```python
from build123d import *

# Parameters (mm, degrees)
SWEEP3_PROFILE_R    = 3.1
SKETCH17_R          = 4.95
BOSS_EXTRUDE1_DEPTH = 15
SKETCH18_R          = 3.85
BOSS_EXTRUDE2_DEPTH = 5
SKETCH19_R          = 4.95
BOSS_EXTRUDE3_DEPTH = 15
SKETCH20_R          = 3.85
BOSS_EXTRUDE4_DEPTH = 5


with BuildPart() as part:
    # Sweep3: sweep along a path in Sketch9
    with BuildLine(Plane.XY) as sweep3_path:
        Line((-183.399133976, 40), (-183.399133976, 180))
        ThreePointArc((-183.399133976, 180), (-130.108654619, 241.593132461), (-61.492979679, 197.712860026))
    # Sweep3 profile (on start of the path) → Sweep3 (sweep)
    with BuildSketch(Plane(origin=(-183.399133976, 40, 0), x_dir=(0, 0, 1), z_dir=(0, 1, 0))):
        Circle(SWEEP3_PROFILE_R)
    sweep(path=sweep3_path.line)

    # Sketch17 → Boss-Extrude1 (add)
    with BuildSketch(Plane.XZ.offset(-40)):
        with Locations((-183.399133976, 0)):
            Circle(SKETCH17_R)
    extrude(amount=BOSS_EXTRUDE1_DEPTH)

    # Sketch18 → Boss-Extrude2 (add)
    with BuildSketch(Plane.XZ.offset(-25)):
        with Locations((-183.399133976, 0)):
            Circle(SKETCH18_R)
    extrude(amount=BOSS_EXTRUDE2_DEPTH)

    # Sketch19 → Boss-Extrude3 (add)
    with BuildSketch(Plane(origin=(-58.920841531, 198.476439545, 0), x_dir=(0.9586493060523679, 0.28459007011017384, 0), z_dir=(0.2845900701101738, -0.9586493060523678, 0))):
        with Locations(Location((-2.6830856, 0, 0), (0, 0, 180))):
            Circle(SKETCH19_R)
    extrude(amount=BOSS_EXTRUDE3_DEPTH)

    # Sketch20 → Boss-Extrude4 (add)
    with BuildSketch(Plane(origin=(-54.651990479, 184.096699954, 0), x_dir=(0.9586493060523679, 0.2845900701101739, 0), z_dir=(0.28459007011017384, -0.9586493060523678, 0))):
        with Locations(Location((-2.6830856, 0, 0), (0, 0, 180))):
            Circle(SKETCH20_R)
    extrude(amount=BOSS_EXTRUDE4_DEPTH)


solid = part.part
```
Here's how the part is built. I have some questions about the finished solid (model axes, mm). A direction names the side the tool comes from. Coordinates: 2 decimals unless noted, no trailing zeros. Order: outer loops, then holes, each group sorted by start corner. A loop starts at its lowest first (then second) coordinate and runs counter-clockwise, first axis right, second up. Notation, with made-up numbers: M -13.75,46.25 L 5.25,46.25 A21 cw 5.25,77.25 Z; hole C -3,-17.5 d3. An arc over 180 degrees is marked long. Answer as a JSON object with one key per item and string values. Group by question number.
(1) If we mould it in two halves opening along X, with no side actions, what happens to faces 1 (the face through (-52.835, 182.065, -0.169)), 2 (the face through (-183, 20, 0)), 3 (the face through (-187.245, 22.535, 0.169))? For each: released by +X, released by -X, zero draft, split by the parting line, or undercut.
(2) For pin 1 (2 mm diameter, centred on x = -174.5, y = 216, fed in from -Z), with a flat end and sliding along its axis, tell me the tip position at first contact or that it passes through.
(3) Which directions (+Z, -Z, +X, -X, +Y, -Y) give clear straight access to the entire face, cutting with the end or side of a thin tool? Please do faces 4 (the face through (-188.344, 32.605, 0.218)), 5 (the face through (-57.2, 183.34, 4.01)), 6 (the face through (-55.75, 178.555, -0.054)).
(4) Suppose I cut it at A-A, the plane z = 0. Please give me the cut outline in (x, y).
(5) I need wall thicknesses on probe 1 along X at (y, z) = (81.5, 0.5); probe 2 along X at (y, z) = (204, 2.25); probe 3 along X at (y, z) = (217.5, 2). Which ranges of each line are inside material? Lowest first, please.
(6) Suppose I cut it at B-B, the plane y = 163. Please give me the cut outline in (x, z), then the cut area to 3 significant figures.
Values found:
{
 "1": {"face 1": "undercut", "face 2": "zero draft", "face 3": "split by the parting line"},
 "2": {"pin 1": "stops at z = -2.89"},
 "3": {"face 4": "-Y", "face 5": "none", "face 6": "+Z, -Z, +X, -Y"},
 "4": {"outline": "M -188.35,25 L -187.25,25 L -187.25,20 L -179.55,20 L -179.55,25 L -178.45,25 L -178.45,40 L -180.3,40 L -180.3,180 A59.14 cw -64.46,196.83 L -66.24,196.3 L -61.97,181.92 L -60.91,182.24 L -59.49,177.44 L -52.11,179.64 L -53.53,184.43 L -52.48,184.74 L -56.75,199.12 L -58.52,198.6 A65.34 ccw -186.5,180 L -186.5,40 L -188.35,40 Z"},
 "5": {"probe 1": "x = -186.46 to -180.34", "probe 2": "x = -180.89 to -176.27, -66.05 to -61.43", "probe 3": "x = -173.77 to -167.83, -74.49 to -68.55"},
 "6": {"outline": "C -183.4,0 d6.2", "area": "30.2 mm^2"}
}
